```python
from build123d import *

# Parameters (mm, degrees)
SALIENTE_EXTRUIR1_DEPTH = 50
CROQUIS2_R              = 7.5
SALIENTE_EXTRUIR2_DEPTH = 75
REDONDEO1_R             = 25
REDONDEO2_R             = 5


with BuildPart() as part:
    # Croquis1 → Saliente-Extruir1 (new body)
    with BuildSketch(Plane.XY):
        Polygon((0, 0), (0, 50), (12.5, 50), (12.5, 0), (62.5, 0), (62.5, 50), (75, 50), (75, -12.5), (0, -12.5), align=None)
    extrude(amount=SALIENTE_EXTRUIR1_DEPTH)

    # Croquis2 → Saliente-Extruir2 (add)
    with BuildSketch(Plane(origin=(75, 0, 0), x_dir=(0, 0, -1), z_dir=(1, 0, 0))):
        with Locations(Location((-25, 30, 0), (0, 0, 180))):
            Circle(CROQUIS2_R)
    extrude(amount=-SALIENTE_EXTRUIR2_DEPTH)

    # Redondeo1
    redondeo1_edges = [part.edges().sort_by_distance(p)[0] for p in [
        (6.25, 50, 0),
        (6.25, 50, 50),
        (68.75, 50, 50),
        (68.75, 50, 0),
    ]]
    fillet(redondeo1_edges, radius=REDONDEO1_R - 0.0001)  # a hair under: the kernel refuses the full size

    # Redondeo2
    redondeo2_edges = [part.edges().sort_by_distance(p)[0] for p in [
        (0, 6.25005, 50),
        (0, 6.25005, 0),
        (37.5, 0, 50),
        (62.5, 12.50005, 50),
        (75, 6.25005, 0),
        (12.5, 12.50005, 0),
        (12.5, 12.50005, 50),
        (12.5, 42.677698819, 42.677698819),
        (12.5, 42.677698819, 7.322301181),
        (0, 42.677698819, 42.677698819),
        (0, 42.677698819, 7.322301181),
        (75, 6.25005, 50),
        (75, 42.677698819, 7.322301181),
        (75, 42.677698819, 42.677698819),
        (62.5, 42.677698819, 7.322301181),
        (62.5, 42.677698819, 42.677698819),
        (62.5, 12.50005, 0),
        (37.5, 0, 0),
    ]]
    fillet(redondeo2_edges, radius=REDONDEO2_R)


solid = part.part
```
Design review of the part built by this model. Coordinates are the model's own, in mm. A direction names the side the tool comes from. Round coordinates to 2 decimals unless told otherwise and drop trailing zeros. Order: outer loops, then holes, each group sorted by start corner. A loop starts at its lowest first (then second) coordinate and runs counter-clockwise, first axis right, second up. Notation, with made-up numbers: M 29.5,45.25 L 60.5,45.25 A34 ccw 60.5,76.25 Z; hole C 78.5,15 d9. An arc over 180 degrees is marked long. Put each result on its own line as item: value.
Q1. To check wall thickness, follow line 1 (X direction, y = 3, z = 29); line 2 (Y direction, x = 51.5, z = 12); line 3 (Y direction, x = 49, z = 20). State the ranges of each line that lie inside material, in increasing order.
Reported:
line 1: 0 to 12.5, 62.5 to 75
line 2: -12.5 to 0
line 3: -12.5 to 0, 24.41 to 35.59
Q2. Draft analysis for pull direction Y (two halves, no side actions). For faces 1 (the face through (11, 9.79, 1.43)), 2 (the face through (37.85, 34.564, 19.048)), 3 (the face through (38, -12.5, 25)), state which applies: released by +Y, released by -Y, zero draft, split by the parting line, or undercut.
Reported:
face 1: zero draft
face 2: undercut
face 3: released by -Y
Q3. Consider section A-A (y = 4). State the section outline as (x, z) points, and give its area (3 significant figures).
Reported:
outline: M 0,5 A5 ccw 5,0 L 7.5,0 A5 ccw 12.5,5 L 12.5,45 A5 ccw 7.5,50 L 5,50 A5 ccw 0,45 Z; M 62.5,5 A5 ccw 67.5,0 L 70,0 A5 ccw 75,5 L 75,45 A5 ccw 70,50 L 67.5,50 A5 ccw 62.5,45 Z
area: 1,210 mm²
Q4. Insertion check: pin 1 Ø6 at (x, y) = (21, 36) entering from -Z; pin 2 Ø1.5 at (y, z) = (43.5, 38.5) entering from +X. Each pin has a flat end and moves straight along its axis. Give the tip position at first contact, or say it passes through.
Reported:
pin 1: z = 18.13
pin 2: x = 74.51
Q5. Consider section B-B (x = 50.5). State the section outline as (y, z) points.
Reported:
outline: M -12.5,0 L -5,0 A5 ccw 0,5 L 0,45 A5 ccw -5,50 L -12.5,50 Z; C 30,25 d15
Q6. Machinability: for faces 4 (the face through (37, 0, 25)), 5 (the face through (12.5, 18, 25)), 6 (the face through (38, -2, 1)), 7 (the face through (11, 10.21, 48.57)), which of the approach directions +Z, -Z, +X, -X, +Y, -Y give a long, thin tool a straight path to every point of the face, cutting with its end or side? Answer none if there is none.
Reported:
face 4: +Z, -Z
face 5: none
face 6: -Z, +Y
face 7: +Z, +Y
